Verification items for the finished model (mm, model axes). A direction names the side the tool comes from. Give positions to 0.01 mm unless a question says otherwise; leave off trailing zeros. Write each loop counter-clockwise with the first axis right and the second up, starting at its lowest first coordinate (ties: lowest second). Pieces come first, ordered by that corner, then holes. Notation, with made-up numbers: M 77,-6 L 101,-6 A16 cw 101,13 Z; hole C -15.5,5.25 d7. An arc over 180 degrees is marked long. Write item = value, one per line.
from build123d import *

# Parameters (mm, degrees)
SKETCH1_R           = 6
BOSS_EXTRUDE1_DEPTH = 2
FILLET1_R           = 10


with BuildPart() as part:
    # Sketch1 → Boss-Extrude1 (new body)
    with BuildSketch(Plane.XY):
        with BuildLine():
            ThreePointArc((-6.17544468, 3), (-19.5, 0), (-6.17544468, -3))
            Line((-6.17544468, -3), (6.17544468, -3))
            ThreePointArc((6.17544468, -3), (19.5, 0), (6.17544468, 3))
            Line((6.17544468, 3), (-6.17544468, 3))
        make_face()
        with Locations((-12.5, 0)):
            Circle(SKETCH1_R, mode=Mode.SUBTRACT)
        with Locations((12.5, 0)):
            Circle(SKETCH1_R, mode=Mode.SUBTRACT)
    extrude(amount=BOSS_EXTRUDE1_DEPTH)

    # Fillet1
    fillet1_edges = [part.edges().sort_by_distance(p)[0] for p in [
        (-6.17544468, 3, 1),
        (6.17544468, 3, 1),
        (6.17544468, -3, 1),
        (-6.17544468, -3, 1),
    ]]
    fillet(fillet1_edges, radius=FILLET1_R)


solid = part.part
1) Draft check along X on faces 1 (the cylindrical face through (19.496, -0.223, 0.986)), 2 (the flat face through (0, 0, 2)). Enter one of: +X half, -X half, draft (parallel to the pull), parting line (faces both ways), or undercut.
From the geometry:
face_1 = undercut
face_2 = draft
2) Cross-section at C-C on x = -12.5. Record the boundary of the cut face in (y, z).
From the geometry:
outline = M -7,0 L -6,0 L -6,2 L -7,2 Z; M 6,0 L 7,0 L 7,2 L 6,2 Z
3) Cross-section at D-D on y = -4.5. Record the boundary of the cut face in (x, z).
From the geometry:
outline = M -17.86,0 L -16.47,0 L -16.47,2 L -17.86,2 Z; M -8.53,0 L -6.81,0 L -6.81,2 L -8.53,2 Z; M 6.81,0 L 8.53,0 L 8.53,2 L 6.81,2 Z; M 16.47,0 L 17.86,0 L 17.86,2 L 16.47,2 Z
4) Cross-section at A-A on z = 0.95. Record the boundary of the cut face in (x, y), plus the area to 3 significant figures.
From the geometry:
outline = M -7.99,-5.35 A10 cw -1.55,-3 L 1.55,-3 A10 cw 7.99,-5.35 A7 ccw long 7.99,5.35 A10 cw 1.55,3 L -1.55,3 A10 cw -7.99,5.35 A7 ccw long Z; hole C -12.5,0 d12; hole C 12.5,0 d12
area = 160 mm^2
5) Cross-section at B-B on y = 0. Record the boundary of the cut face in (x, z).
From the geometry:
outline = M -19.5,0 L -18.5,0 L -18.5,2 L -19.5,2 Z; M -6.5,0 L 6.5,0 L 6.5,2 L -6.5,2 Z; M 18.5,0 L 19.5,0 L 19.5,2 L 18.5,2 Z
6) Material ranges on probe 1 along Y at (x, z) = (-12.5, 1.55); probe 2 along X at (y, z) = (2, 0.65); probe 3 along X at (y, z) = (0.5, 0.45), recorded low to high. Write a range as from..to.
From the geometry:
probe_1 = -7..-6, 6..7
probe_2 = -19.21..-18.16, -6.84..6.84, 18.16..19.21
probe_3 = -19.48..-18.48, -6.52..6.52, 18.48..19.48
7) Tool access check on faces 3 (the cylindrical face through (-5.022, -3.624, 1.014)), 4 (the cylindrical face through (4.93, 3.59, 1.01)), 5 (the cylindrical face through (-19.496, 0.223, 0.986)). Record the directions out of +Z, -Z, +X, -X, +Y, -Y that give a thin tool (end or side, any length) a straight path to the whole face; none if there is none.
From the geometry:
face_3 = +Z, -Z, -Y
face_4 = +Z, -Z, +Y
face_5 = +Z, -Z
8) Depth check by flat-ended pin: P1, Ø0.6, axis at x = 0, z = 1.5, coming from the +Y side. Enter the tip coordinate at first touch or a pass-through.
From the geometry:
P1 = 3
